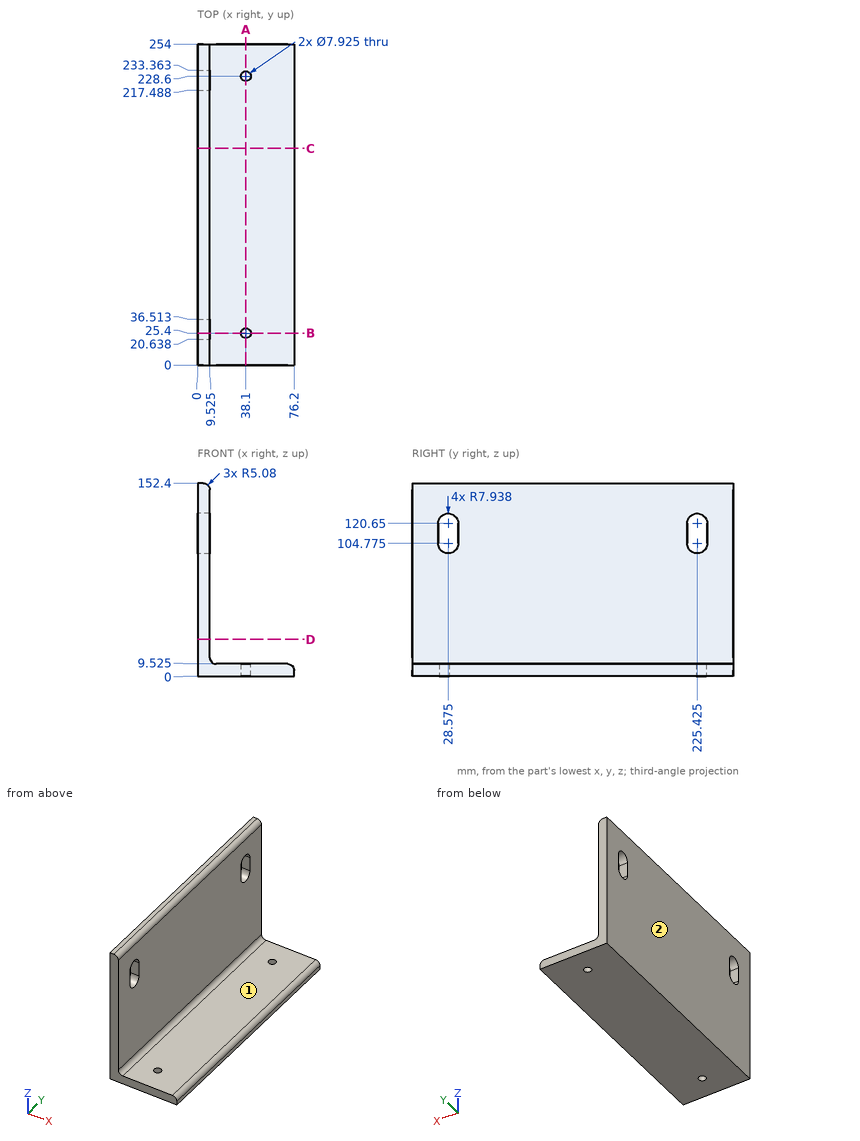
Print and shaded views of the part. All mm, measured from the part's lowest x, y and z. A direction names the side the tool comes from. Give positions to 0.01 mm unless a question says otherwise; leave off trailing zeros. Write each loop counter-clockwise with the first axis right and the second up, starting at its lowest first coordinate (ties: lowest second). Pieces come first, ordered by that corner, then holes. Notation, with made-up numbers: (-14, 4.5) - (-8, 4.5) arc R29 ccw to (-8, 34.5) - close; hole circle Ø7 at (83.5, 78.25). An arc over 180 degrees is marked (long way). One line per question, with ' | ' between items. Start each with the question number.
(1) Wall check: line 1 along Y through (x, z) = (38.1, 2.75); line 2 along X through (y, z) = (25, 3); line 3 along X through (y, z) = (228.6, 4.75). Give the ranges that are in metal, low to high. Write a range as from..to.
(2) 3-axis set-ups, long thin cutter, end or side, ignore diameter. For the marked faces 1 and 2: which of +Z, -Z, +X, -X, +Y, -Y reach the whole face in a straight line?
(3) Slice it at C-C on y = 171.5. Write the cut outline in (x, z) (1 decimal).
(4) Pin check, flat tips, straight feed: P1, Ø2, axis at x = 20.5, y = 179, coming from the +Z side (1 decimal); P2, Ø6, axis at y = 131, z = 99.5, coming from the +X side (1 decimal); P3, Ø6, axis at x = 17, y = 206.5, coming from the +Z side. Stop position of each tip, or through.
(5) Slice it at B-B on y = 25.4. Write the cut outline in (x, z) (1 decimal).
(6) Slice it at D-D on z = 29. Write the cut outline in (x, y) (1 decimal).
(7) Slice it at A-A on x = 38.1. Write the cut outline in (y, z) (1 decimal).
Results below:
1) line 1: 0..21.44, 29.36..224.64, 232.56..254 | line 2: 0..34.16, 42.04..76.2 | line 3: 0..34.14, 42.06..76.19
2) face 1: +Z, +X, +Y, -Y | face 2: +Z, -Z, -X, +Y, -Y
3) outline: (0, 0) - (76.2, 0) - (76.2, 4.4) arc R5.1 ccw to (71.1, 9.5) - (14.6, 9.5) arc R5.1 cw to (9.5, 14.6) - (9.5, 147.3) arc R5.1 ccw to (4.4, 152.4) - (0, 152.4) - close
4) P1: z = 9.5 | P2: x = 9.5 | P3: z = 9.56
5) outline: (0, 0) - (34.1, 0) - (34.1, 9.5) - (14.6, 9.5) arc R5.1 cw to (9.5, 14.6) - (9.5, 97.5) - (0, 97.5) - close; (0, 127.9) - (9.5, 127.9) - (9.5, 147.3) arc R5.1 ccw to (4.4, 152.4) - (0, 152.4) - close; (42.1, 0) - (76.2, 0) - (76.2, 4.4) arc R5.1 ccw to (71.1, 9.5) - (42.1, 9.5) - close
6) outline: (0, 0) - (9.5, 0) - (9.5, 254) - (0, 254) - close
7) outline: (0, 0) - (21.4, 0) - (21.4, 9.5) - (0, 9.5) - close; (29.4, 0) - (224.6, 0) - (224.6, 9.5) - (29.4, 9.5) - close; (232.6, 0) - (254, 0) - (254, 9.5) - (232.6, 9.5) - close
